CAD build for the part. Positions are in the model's coordinates, mm. A direction names the side the tool comes from. Give positions to 0.01 mm unless a question says otherwise; leave off trailing zeros. Loops run counter-clockwise (first coordinate to the right, second up) from the corner with the lowest first, then second, coordinate; pieces in that order, holes last. Notation, with made-up numbers: (62.5, -31) - (104.5, -31) arc R22 ccw to (104.5, -24) - close; hole circle Ø2 at (74, 1). An arc over 180 degrees is marked (long way). Return JSON: item names as keys, results as strings.
from build123d import *

# Parameters (mm, degrees)
SKETCH_1_R      = 3.85
EXTRUDE_1_DEPTH = 1.5


with BuildPart() as part:
    # 草圖1 → 填料-伸長1 (new body)
    with BuildSketch(Plane(origin=(0, 0, 0), x_dir=(0, 0, -1), z_dir=(1, 0, 0))):
        with BuildLine():
            Line((251.501318297, 74.382976373), (100.201901366, 74.382976373))
            ThreePointArc((100.201901366, 74.382976373), (89.968438713, 72.236892378), (81.459379698, 66.160269216))
            ThreePointArc((81.459379698, 66.160269216), (60.428444362, 64.718846971), (67.717817707, 84.498709848))
            ThreePointArc((67.717817707, 84.498709848), (80.697411325, 86.098517108), (93.764300282, 86.632976373))
            Line((93.764300282, 86.632976373), (249.095497945, 86.632976373))
            Line((249.095497945, 86.632976373), (283.552477777, 86.632976373))
            ThreePointArc((283.552477777, 86.632976373), (295.765347138, 64.159226657), (270.264218528, 66.138126331))
            Line((270.264218528, 66.138126331), (270.243839965, 66.160269216))
            ThreePointArc((270.243839965, 66.160269216), (261.734780949, 72.236892378), (251.501318297, 74.382976373))
        make_face()
        with Locations((70.477225092, 72.248709848)):
            Circle(SKETCH_1_R, mode=Mode.SUBTRACT)
        with Locations((284.227225092, 72.248709848)):
            Circle(SKETCH_1_R, mode=Mode.SUBTRACT)
    extrude(amount=EXTRUDE_1_DEPTH)


solid = part.part
1. Cut at A-A, the plane y = 62.5. Write the cut outline in (x, z), plus the area to 3 significant figures.
Values follow:
{"outline": "(0, -294.51) - (1.5, -294.51) - (1.5, -272.59) - (0, -272.59) - close; (0, -78.39) - (1.5, -78.39) - (1.5, -62.56) - (0, -62.56) - close", "area": "56.6 mm²"}
2. Cut at C-C, the plane z = -133. Write the cut outline in (x, y).
Values follow:
{"outline": "(0, 74.38) - (1.5, 74.38) - (1.5, 86.63) - (0, 86.63) - close"}
3. Drop a flat-ended pin along its axis: P1, Ø0.8, axis at x = 1, z = -167, coming from the -Y side. Give the stop position or say it passes through.
Values follow:
{"P1": "stops at y = 74.38"}
4. Which spindle directions (+Z, -Z, +X, -X, +Y, -Y) get a long thin tool onto all of the face, cutting with end or side? Do faces 1 (the face through (0.74, 72.177, -261.87)), 2 (the face through (0.74, 75.495, -72.547)). Say none if no direction does.
Values follow:
{"face 1": "+X, -X, -Y", "face 2": "+X, -X"}
5. Pull direction Z, two halves, no side cores. Call faces 3 (the face through (0, 79, -180)), 4 (the face through (0.74, 72.296, -90.104)): +Z half, -Z half, draft (parallel to the pull), parting line (faces both ways), or undercut.
Values follow:
{"face 3": "draft", "face 4": "undercut"}
6. Cut at B-B, the plane x = 1. Give the number of separate pieces and of enclosed holes in the cut face, plus the area to 3 significant figures.
Values follow:
{"separate pieces": "1", "enclosed holes": "2", "area": "3,510 mm²"}
7. Cut at D-D, the plane y = 82. Write the cut outline in (x, z).
Values follow:
{"outline": "(0, -294.2) - (1.5, -294.2) - (1.5, -62.57) - (0, -62.57) - close"}
8. Drill centre lines: probe 1 along Z at (x, y) = (0.85, 71); probe 2 along Y at (x, z) = (1, -232); probe 3 along Z at (x, y) = (1.15, 66.5). Where is each one in solid material? Low to high.
Values follow:
{"probe 1": "z = -298.07 to -287.87, -280.59 to -264.19, -87.52 to -74.12, -66.84 to -57.98", "probe 2": "y = 74.38 to 86.63", "probe 3": "z = -297 to -269.93, -81.78 to -59.31"}
